```python
from build123d import *

# Parameters (mm, degrees)
BOSS_EXTRUDE1_DEPTH = 27
SKETCH2_R           = 1.5
BOSS_EXTRUDE2_DEPTH = 3
FILLET1_R           = 1


with BuildPart() as part:
    # Sketch1 → Boss-Extrude1 (new body)
    with BuildSketch(Plane(origin=(0, 64.224437766, -64.224437766), x_dir=(1, 0, 0), z_dir=(0, 0.7071067811865498, -0.7071067811865452))):
        with BuildLine():
            Line((91.844609768, -130.551114539), (88.844609768, -130.551114539))
            ThreePointArc((88.844609768, -130.551114539), (73.844609768, -145.551114539), (58.844609768, -130.551114539))
            Line((58.844609768, -130.551114539), (55.844609768, -130.551114539))
            ThreePointArc((55.844609768, -130.551114539), (73.844609768, -148.551114539), (91.844609768, -130.551114539))
        make_face()
    extrude(amount=-BOSS_EXTRUDE1_DEPTH)

    # Sketch2 → Boss-Extrude2 (add)
    # profile 1 of 2: a face of its own
    with BuildSketch(Plane(origin=(0, 92.313578382, 92.313578382), x_dir=(1, 0, 0), z_dir=(-1.3084103822363938e-14, 0.7071067811865454, 0.7071067811865497))):
        with BuildLine():
            Line((97.77004577, 80.702506927), (88.844609768, 83.149574448))
            Line((88.844609768, 83.149574448), (88.844609768, 71.5045674))
            Line((88.844609768, 71.5045674), (97.77004577, 73.951634922))
            ThreePointArc((97.77004577, 73.951634922), (100.344609768, 77.327070924), (97.77004577, 80.702506927))
        make_face()
        with Locations(Location((96.844609768, 77.327070924, 0), (0, 0, 270))):
            Circle(SKETCH2_R, mode=Mode.SUBTRACT)
    # profile 2 of 2: a face of its own
    with BuildSketch(Plane(origin=(0, 92.313578382, 92.313578382), x_dir=(1, 0, 0), z_dir=(-1.3084103822363938e-14, 0.7071067811865454, 0.7071067811865497))):
        with BuildLine():
            Line((49.919173765, 73.951634922), (58.844609768, 71.5045674))
            Line((58.844609768, 71.5045674), (58.844609768, 83.149574448))
            Line((58.844609768, 83.149574448), (49.919173765, 80.702506927))
            ThreePointArc((49.919173765, 80.702506927), (47.344609768, 77.327070924), (49.919173765, 73.951634922))
        make_face()
        with Locations(Location((50.844609768, 77.327070924, 0), (0, 0, 270))):
            Circle(SKETCH2_R, mode=Mode.SUBTRACT)
    extrude(amount=BOSS_EXTRUDE2_DEPTH)

    # Fillet1
    fillet1_edges = [part.edges().sort_by_distance(p)[0] for p in [
        (91.592849117, 149.113394945, 39.756402505),
        (56.096370418, 149.113394945, 39.756402505),
    ]]
    fillet(fillet1_edges, radius=FILLET1_R)


solid = part.part
```
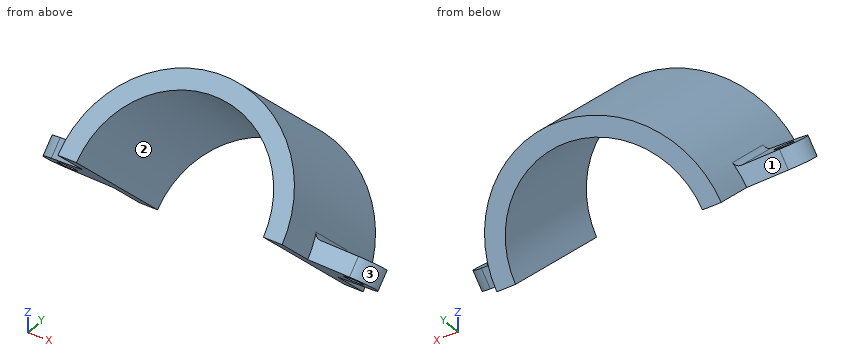
The model under review builds one solid part; all positions refer to its coordinate system, in mm. Face numbers are marked on the shaded views. Give positions to 0.01 mm unless a question says otherwise; leave off trailing zeros. Write each loop counter-clockwise with the first axis right and the second up, starting at its lowest first coordinate (ties: lowest second). Pieces come first, ordered by that corner, then holes. Notation, with made-up numbers: M -20,86 L 1,86 A29 cw 1,123 Z; hole C 59,-16 d3. An arc over 180 degrees is marked long. Answer in a Markdown table with one row per item.
Item 1: Draft analysis for pull direction X (two halves, no side actions). For the marked faces 1, 2 and 3, state which applies: +X half, -X half, draft (parallel to the pull), parting line (faces both ways), or undercut.
Check sheet entries:
| item | result |
|---|---|
| face 1 | -X half |
| face 2 | undercut |
| face 3 | +X half |
Item 2: Add section B-B on x = 61. Give the boundary of the cut face in (y, z).
Check sheet entries:
| item | result |
|---|---|
| outline | M 142.92,52.66 L 162.02,33.57 L 165.45,37.01 L 146.36,56.1 Z |
Item 3: Add section A-A on x = 68. Give the boundary of the cut face in (y, z).
Check sheet entries:
| item | result |
|---|---|
| outline | M 147.21,56.95 L 166.31,37.86 L 168.58,40.13 L 149.48,59.22 Z |
Item 4: For line 1 along X through (y, z) = (145, 44); line 2 along X through (y, z) = (145, 49.5); line 3 along Y through (x, z) = (79, 56.5), list the stretches that pass through material, from the lowest coordinate up.
Check sheet entries:
| item | result |
|---|---|
| line 1 | 56.11 to 59.17, 88.52 to 91.58 |
| line 2 | 57.25 to 60.57, 87.12 to 90.44 |
| line 3 | 148.05 to 152.52 |
Item 5: For P1, Ø8, axis at y = 157.5, z = 45, coming from the -X side; P2, Ø5, axis at x = 74, y = 151.5, coming from the -Z side; P3, Ø1, axis at x = 60.5, y = 147.5, coming from the +Z side, all flat-tipped, find the tip position at first contact; note any pin that passes through.
Check sheet entries:
| item | result |
|---|---|
| P1 | x = 58.05 |
| P2 | z = 51.84 |
| P3 | z = 55.12 |
